Part model, mm, in its own coordinate system. Face numbers are marked on the shaded views. A direction names the side the tool comes from. Give positions to 0.01 mm unless a question says otherwise; leave off trailing zeros. Order: outer loops, then holes, each group sorted by start corner. A loop starts at its lowest first (then second) coordinate and runs counter-clockwise, first axis right, second up. Notation, with made-up numbers: (-35.75, 18.5) - (-23.75, 18.5) arc R17 ccw to (-23.75, 41.5) - close; hole circle Ø3 at (2.25, -40). An arc over 180 degrees is marked (long way). Use one line per item in the form item = value. Start each with the question number.
1. Band-saw the part on D-D, the plane z = -1. List the corners of the cut face in (x, y), plus the area to 3 significant figures.
2. Band-saw the part on C-C, the plane x = -4.5. State how many separate pieces and enclosed holes the cut face has, plus the area to 3 significant figures.
3. Tool access for the marked faces 4, 5 and 6: list every direction of +Z, -Z, +X, -X, +Y, -Y with a clear straight run to the whole face (end or side of a thin tool).
4. Drill centre lines: line 1 (X direction, y = 0, z = 6); line 2 (X direction, y = 39.5, z = 6.75); line 3 (Y direction, x = 3.85, z = 5). Where is each one in solid material? Low to high.
5. Band-saw the part on A-A, the plane z = 9. List the corners of the cut face in (x, y), plus the area to 3 significant figures.
6. Pull direction Y, two halves, no side cores. Call the marked faces 1, 2 and 3: +Y half, -Y half, draft (parallel to the pull), parting line (faces both ways), or undercut.
7. Pin check, flat tips, straight feed: P1, Ø6.5, axis at y = -24.5, z = 3, coming from the +X side; P2, Ø1.1, axis at x = 9, z = 8, coming from the -Y side; P3, Ø2.5, axis at x = 0, y = 41.5, coming from the -Z side. Stop position of each tip, or through.
8. Band-saw the part on B-B, the plane y = 32. List the corners of the cut face in (x, z), plus the area to 3 significant figures.
Autodesk Fusion 360 part; units mm, degrees
ref_plane "工作平面1" through (0, 0, 0) normal (0, 0, 1) x (1, 0, 0)
sketch "草图1" plane through (0, 0, 0) normal (0, 0, 1) x (1, 0, 0)
  line L0 (-26, -22) -> (26, -22)
  line L1 (26, -22) -> (28, -20)
  line L2 (28, -20) -> (28, 20)
  line L3 (28, 20) -> (26, 22)
  line L4 (26, 22) -> (-26, 22)
  line L5 (-26, 22) -> (-28, 20)
  line L6 (-28, 20) -> (-28, -20)
  line L7 (-28, -20) -> (-26, -22)
extrude "56 x 44 x 7 platform" add sketch "草图1" along normal blind 12
ref_plane "工作平面2" through (0, 0, 12) normal (0, 0, 1) x (1, 0, 0)
sketch "草图2" plane through (0, 0, 12) normal (0, 0, 1) x (1, 0, 0)
  line L0 (-28, -22) -> (-20.49, -22)
  line L1 (-20.49, -22) -> (-20.49, 22)
  line L2 (-20.49, 22) -> (-28, 22)
  line L3 (-28, 22) -> (-28, -22)
ref_plane "工作平面3" through (0, 0, 17.2) normal (0, 0, 1) x (1, 0, 0)
sketch "草图3" plane through (0, 0, 17.2) normal (0, 0, 1) x (1, 0, 0)
  line L0 (-28, -22) -> (-16.33, -22)
  line L1 (-16.33, -22) -> (-16.33, 22)
  line L2 (-16.33, 22) -> (-28, 22)
  line L3 (-28, 22) -> (-28, -22)
loft "Dovetail retaining rail 0.8 to 1 -1" add profiles "草图2", "草图3" section 1 section 2
ref_plane "工作平面4" through (0, 0, 11.7) normal (0, 0, 1) x (1, 0, 0)
sketch "草图4" plane through (0, 0, 11.7) normal (0, 0, 1) x (1, 0, 0)
  line L0 (-23.4, -22) -> (-22.5, -22)
  line L1 (-22.5, -22) -> (-22.5, 13)
  line L2 (-22.5, 13) -> (-23.4, 13)
  line L3 (-23.4, 13) -> (-23.4, -22)
extrude "0.9 mm longitudinal flexure slot -1" cut sketch "草图4" along normal blind 5.8
ref_plane "工作平面5" through (0, 0, 11.7) normal (0, 0, 1) x (1, 0, 0)
sketch "草图5" plane through (0, 0, 11.7) normal (0, 0, 1) x (1, 0, 0)
  line L0 (-22.5, -22) -> (-15, -22)
  line L1 (-15, -22) -> (-15, 13)
  line L2 (-15, 13) -> (-22.5, 13)
  line L3 (-22.5, 13) -> (-22.5, -22)
extrude "0.8 mm flexure underside relief -1" cut sketch "草图5" along normal blind 0.8
ref_plane "工作平面6" through (0, 0, 12.6) normal (0, 0, 1) x (1, 0, 0)
sketch "草图6" plane through (0, 0, 12.6) normal (0, 0, 1) x (1, 0, 0)
  line L0 (-20.21, -6) -> (-20.21, 11)
  line L1 (-20.21, 11) -> (-19.66, 11)
  line L2 (-19.66, 11) -> (-19.66, 2)
  line L3 (-19.66, 2) -> (-20.11, -6)
  line L4 (-20.11, -6) -> (-20.21, -6)
ref_plane "工作平面7" through (0, 0, 16.8) normal (0, 0, 1) x (1, 0, 0)
sketch "草图7" plane through (0, 0, 16.8) normal (0, 0, 1) x (1, 0, 0)
  line L0 (-16.85, -6) -> (-16.85, 11)
  line L1 (-16.85, 11) -> (-16.3, 11)
  line L2 (-16.3, 11) -> (-16.3, 2)
  line L3 (-16.3, 2) -> (-16.75, -6)
  line L4 (-16.75, -6) -> (-16.85, -6)
loft "Tapered friction contact rib -1" add profiles "草图6", "草图7" section 1 section 2
ref_plane "工作平面8" through (0, 0, 12) normal (0, 0, 1) x (1, 0, 0)
sketch "草图8" plane through (0, 0, 12) normal (0, 0, 1) x (1, 0, 0)
  line L0 (20.49, -22) -> (28, -22)
  line L1 (28, -22) -> (28, 22)
  line L2 (28, 22) -> (20.49, 22)
  line L3 (20.49, 22) -> (20.49, -22)
ref_plane "工作平面9" through (0, 0, 17.2) normal (0, 0, 1) x (1, 0, 0)
sketch "草图9" plane through (0, 0, 17.2) normal (0, 0, 1) x (1, 0, 0)
  line L0 (16.33, -22) -> (28, -22)
  line L1 (28, -22) -> (28, 22)
  line L2 (28, 22) -> (16.33, 22)
  line L3 (16.33, 22) -> (16.33, -22)
loft "Dovetail retaining rail 0.8 to 1 1" add profiles "草图8", "草图9" section 1 section 2
ref_plane "工作平面10" through (0, 0, 11.7) normal (0, 0, 1) x (1, 0, 0)
sketch "草图10" plane through (0, 0, 11.7) normal (0, 0, 1) x (1, 0, 0)
  line L0 (22.5, -22) -> (23.4, -22)
  line L1 (23.4, -22) -> (23.4, 13)
  line L2 (23.4, 13) -> (22.5, 13)
  line L3 (22.5, 13) -> (22.5, -22)
extrude "0.9 mm longitudinal flexure slot 1" cut sketch "草图10" along normal blind 5.8
ref_plane "工作平面11" through (0, 0, 11.7) normal (0, 0, 1) x (1, 0, 0)
sketch "草图11" plane through (0, 0, 11.7) normal (0, 0, 1) x (1, 0, 0)
  line L0 (15, -22) -> (22.5, -22)
  line L1 (22.5, -22) -> (22.5, 13)
  line L2 (22.5, 13) -> (15, 13)
  line L3 (15, 13) -> (15, -22)
extrude "0.8 mm flexure underside relief 1" cut sketch "草图11" along normal blind 0.8
ref_plane "工作平面12" through (0, 0, 12.6) normal (0, 0, 1) x (1, 0, 0)
sketch "草图12" plane through (0, 0, 12.6) normal (0, 0, 1) x (1, 0, 0)
  line L0 (20.21, -6) -> (20.21, 11)
  line L1 (20.21, 11) -> (19.66, 11)
  line L2 (19.66, 11) -> (19.66, 2)
  line L3 (19.66, 2) -> (20.11, -6)
  line L4 (20.11, -6) -> (20.21, -6)
ref_plane "工作平面13" through (0, 0, 16.8) normal (0, 0, 1) x (1, 0, 0)
sketch "草图13" plane through (0, 0, 16.8) normal (0, 0, 1) x (1, 0, 0)
  line L0 (16.85, -6) -> (16.85, 11)
  line L1 (16.85, 11) -> (16.3, 11)
  line L2 (16.3, 11) -> (16.3, 2)
  line L3 (16.3, 2) -> (16.75, -6)
  line L4 (16.75, -6) -> (16.85, -6)
loft "Tapered friction contact rib 1" add profiles "草图12", "草图13" section 1 section 2
ref_plane "工作平面14" through (0, 0, 12) normal (0, 0, 1) x (1, 0, 0)
sketch "草图14" plane through (0, 0, 12) normal (0, 0, 1) x (1, 0, 0)
  line L0 (-16.5, 19.4) -> (16.5, 19.4)
  line L1 (16.5, 19.4) -> (16.5, 22)
  line L2 (16.5, 22) -> (-16.5, 22)
  line L3 (-16.5, 22) -> (-16.5, 19.4)
extrude "Closed insertion end stop" add sketch "草图14" along normal blind 5.2
ref_plane "工作平面15" through (0, 0, 0) normal (0, 0, 1) x (1, 0, 0)
sketch "草图15" plane through (0, 0, 0) normal (0, 0, 1) x (1, 0, 0)
  circle A0 centre (0, 0) radius 7.5
extrude "15 mm screw and driver access" cut sketch "草图15" along normal blind 12
move_body "Align camera long edge with gimbal arm - 90 degrees" bodies 1 to x (0, 1, 0) y (-1, 0, 0) z (0, 0, 1) at (0, 0, 0)
ref_plane "工作平面16" through (0, 0, 0) normal (0, 0, 1) x (1, 0, 0)
sketch "草图16" plane through (0, 0, 0) normal (0, 0, 1) x (1, 0, 0)
  line L0 (7.8, 5.95) -> (11.4, 5.95)
  line L1 (11.4, 5.95) -> (11.4, 21.05)
  line L2 (11.4, 21.05) -> (7.8, 21.05)
  line L3 (7.8, 21.05) -> (7.8, 5.95)
extrude "Clear original raised tab and root fillet" cut sketch "草图16" along normal blind 11.9
ref_plane "工作平面17" through (0, 0, -2.1) normal (0, 0, 1) x (1, 0, 0)
sketch "草图17" plane through (0, 0, -2.1) normal (0, 0, 1) x (1, 0, 0)
  line L0 (-8.5, -20) -> (-6.3, -20)
  line L1 (-6.3, -20) -> (-6.3, 20)
  line L2 (-6.3, 20) -> (-8.5, 20)
  line L3 (-8.5, 20) -> (-8.5, -20)
extrude "Arm lateral locating shoulder" add sketch "草图17" along normal blind 2.1
ref_plane "工作平面18" through (0, 0, -2.1) normal (0, 0, 1) x (1, 0, 0)
sketch "草图18" plane through (0, 0, -2.1) normal (0, 0, 1) x (1, 0, 0)
  line L0 (8.3, -20) -> (10.5, -20)
  line L1 (10.5, -20) -> (10.5, 20)
  line L2 (10.5, 20) -> (8.3, 20)
  line L3 (8.3, 20) -> (8.3, -20)
extrude "Arm lateral locating shoulder (1)" add sketch "草图18" along normal blind 2.1
ref_plane "工作平面19" through (0, 0, 0) normal (0, 0, 1) x (1, 0, 0)
sketch "草图19" plane through (0, 0, 0) normal (0, 0, 1) x (1, 0, 0)
  circle A0 centre (0, -20) radius 1.2
extrude "M2 through clearance at y -20.0" cut sketch "草图19" along normal blind 12
ref_plane "工作平面20" through (0, 0, 10.3) normal (0, 0, 1) x (1, 0, 0)
sketch "草图20" plane through (0, 0, 10.3) normal (0, 0, 1) x (1, 0, 0)
  circle A0 centre (0, -20) radius 2.25
extrude "M2 head recess at y -20.0" cut sketch "草图20" along normal blind 1.7
ref_plane "工作平面21" through (0, 0, 0) normal (0, 0, 1) x (1, 0, 0)
sketch "草图21" plane through (0, 0, 0) normal (0, 0, 1) x (1, 0, 0)
  circle A0 centre (0, 12) radius 1.2
extrude "M2 through clearance at y 12.0" cut sketch "草图21" along normal blind 12
ref_plane "工作平面22" through (0, 0, 10.3) normal (0, 0, 1) x (1, 0, 0)
sketch "草图22" plane through (0, 0, 10.3) normal (0, 0, 1) x (1, 0, 0)
  circle A0 centre (0, 12) radius 2.25
extrude "M2 head recess at y 12.0" cut sketch "草图22" along normal blind 1.7
ref_plane "工作平面23" through (0, 0, 0) normal (0, 0, 1) x (1, 0, 0)
sketch "草图23" plane through (0, 0, 0) normal (0, 0, 1) x (1, 0, 0)
  line L0 (5, -52.15) -> (8.7, -52.15)
  line L1 (8.7, -52.15) -> (8.7, -27.5)
  line L2 (8.7, -27.5) -> (5, -27.5)
  line L3 (5, -27.5) -> (5, -52.15)
extrude "Ear for original 3.2 mm side hole at arm y -28.15" add sketch "草图23" along normal blind 7.2
ref_plane "工作平面24" through (0, 0, 0) normal (0, 0, 1) x (1, 0, 0)
sketch "草图24" plane through (0, 0, 0) normal (0, 0, 1) x (1, 0, 0)
  line L0 (7.8, -52.15) -> (8.9, -52.15)
  line L1 (8.9, -52.15) -> (8.9, -27.5)
  line L2 (8.9, -27.5) -> (7.8, -27.5)
  line L3 (7.8, -27.5) -> (7.8, -52.15)
extrude "Ear relief around original arm root radius" cut sketch "草图24" along normal blind 1.3
ref_plane "工作平面25" through (4.9, 0, 0) normal (1, 0, 0) x (0, 1, 0)
sketch "草图25" plane through (4.9, 0, 0) normal (1, 0, 0) x (0, 0, -1)
  circle A0 centre (-5, -48.15) radius 1.6
extrude "Side rivet full passage clearance" cut sketch "草图25" along normal blind 20
ref_plane "工作平面26" through (2.9, 0, 0) normal (1, 0, 0) x (0, 1, 0)
sketch "草图26" plane through (2.9, 0, 0) normal (1, 0, 0) x (0, 0, -1)
  circle A0 centre (-5, -48.15) radius 2.9
extrude "Side rivet flange counterbore" cut sketch "草图26" along normal blind 2.2
ref_plane "工作平面27" through (0, 0, 0) normal (0, 0, 1) x (1, 0, 0)
sketch "草图27" plane through (0, 0, 0) normal (0, 0, 1) x (1, 0, 0)
  line L0 (5, 12.85) -> (8.7, 12.85)
  line L1 (8.7, 12.85) -> (8.7, 20.85)
  line L2 (8.7, 20.85) -> (5, 20.85)
  line L3 (5, 20.85) -> (5, 12.85)
extrude "Ear for original 3.2 mm side hole at arm y 36.85" add sketch "草图27" along normal blind 7.2
ref_plane "工作平面28" through (0, 0, 0) normal (0, 0, 1) x (1, 0, 0)
sketch "草图28" plane through (0, 0, 0) normal (0, 0, 1) x (1, 0, 0)
  line L0 (7.8, 12.85) -> (8.9, 12.85)
  line L1 (8.9, 12.85) -> (8.9, 20.85)
  line L2 (8.9, 20.85) -> (7.8, 20.85)
  line L3 (7.8, 20.85) -> (7.8, 12.85)
extrude "Ear relief around original arm root radius (1)" cut sketch "草图28" along normal blind 1.3
ref_plane "工作平面29" through (4.9, 0, 0) normal (1, 0, 0) x (0, 1, 0)
sketch "草图29" plane through (4.9, 0, 0) normal (1, 0, 0) x (0, 0, -1)
  circle A0 centre (-5, 16.85) radius 1.6
extrude "Side rivet full passage clearance (1)" cut sketch "草图29" along normal blind 20
ref_plane "工作平面30" through (2.9, 0, 0) normal (1, 0, 0) x (0, 1, 0)
sketch "草图30" plane through (2.9, 0, 0) normal (1, 0, 0) x (0, 0, -1)
  circle A0 centre (-5, 16.85) radius 2.9
extrude "Side rivet flange counterbore (1)" cut sketch "草图30" along normal blind 2.2
move_body "Move outward toward free end 20.0 mm" bodies 1 to x (1, 0, 0) y (0, 1, 0) z (0, 0, 1) at (0, 20, 0)
ref_plane "工作平面31" through (0, 0, -2.11) normal (0, 0, 1) x (1, 0, 0)
sketch "草图31" plane through (0, 0, -2.11) normal (0, 0, 1) x (1, 0, 0)
  line L0 (8.29, 25.95) -> (10.51, 25.95)
  line L1 (10.51, 25.95) -> (10.51, 40.05)
  line L2 (10.51, 40.05) -> (8.29, 40.05)
  line L3 (8.29, 40.05) -> (8.29, 25.95)
extrude "Trim locating shoulder before raised side ear root" cut sketch "草图31" along normal blind 2.11
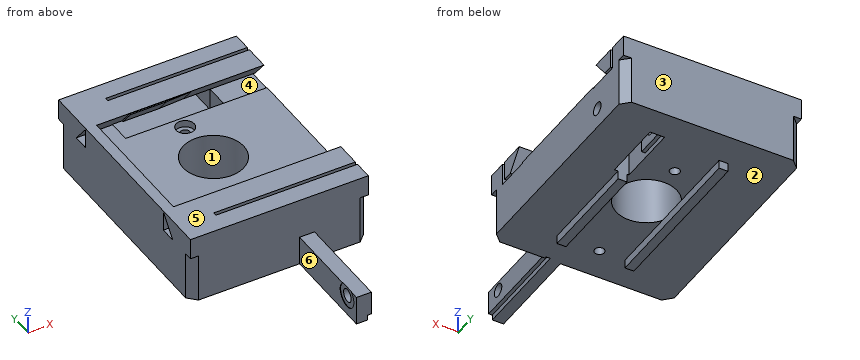
From the geometry:
q1.outline = (-8.5, 0) - (-6.3, 0) - (-6.3, 40) - (-8.5, 40) - close; (8.3, 0) - (10.5, 0) - (10.5, 25.95) - (8.3, 25.95) - close
q1.area = 145 mm²
q2.separate_pieces = 4
q2.enclosed_holes = 0
q2.area = 614 mm²
q3.face_4 = +X
q3.face_5 = +Z, +X, -X, +Y, -Y
q3.face_6 = +Z, -Z, -X, -Y
q4.line_1 = -22 to -1.2, 1.2 to 22
q4.line_2 = -22 to 8.7, 11.4 to 22
q4.line_3 = -8 to 13.56, 26.44 to 33.95, 39.75 to 48
q5.outline = (-22, -6) - (-20, -8) - (20, -8) - (22, -6) - (22, 46) - (20, 48) - (-20, 48) - (-22, 46) - close; hole circle Ø15 at (0, 20); hole circle Ø2.4 at (0, 0); hole circle Ø2.4 at (0, 32); hole (7.8, 25.95) - (11.4, 25.95) - (11.4, 41.05) - (7.8, 41.05) - close
q5.area = 2,220 mm²
q6.face_1 = undercut
q6.face_2 = draft
q6.face_3 = +Y half
q7.P1 = 8.7
q7.P2 = -8
q7.P3 = 0
q8.outline = (-22, 0) - (-8.5, 0) - (-8.5, -2.1) - (-6.3, -2.1) - (-6.3, 0) - (-1.2, 0) - (-1.2, 10.3) - (-2.25, 10.3) - (-2.25, 12) - (-19.4, 12) - (-19.4, 17.2) - (-22, 17.2) - close; (1.2, 0) - (7.8, 0) - (7.8, 11.9) - (11.4, 11.9) - (11.4, 0) - (22, 0) - (22, 12) - (2.25, 12) - (2.25, 10.3) - (1.2, 10.3) - close
q8.area = 471 mm²
